from build123d import *

# Parameters (mm, degrees)
SZKIC1_W                    = 80
SZKIC1_H                    = 65
DODANIE_WYCI_GNI_CIE1_DEPTH = 30
SZKIC2_R                    = 27.5
WYTNIJ_WYCI_GNI_CIE1_DEPTH  = 30
SZKIC4_R                    = 3
WYTNIJ_WYCI_GNI_CIE2_DEPTH  = 30
SFAZOWANIE1_SIZE            = 15
SZKIC6_R                    = 3
WYTNIJ_WYCI_GNI_CIE3_DEPTH  = 25
SZKIC8_R                    = 5
WYTNIJ_WYCI_GNI_CIE5_DEPTH  = 6


with BuildPart() as part:
    # Szkic1 → Dodanie-wyciągnięcie1 (new body)
    with BuildSketch(Plane.XY):
        Rectangle(SZKIC1_W, SZKIC1_H)
    extrude(amount=DODANIE_WYCI_GNI_CIE1_DEPTH)

    # Szkic2 → Wytnij-wyciągnięcie1 (cut)
    with BuildSketch(Plane.XY.offset(30)):
        Circle(SZKIC2_R)
    extrude(amount=-WYTNIJ_WYCI_GNI_CIE1_DEPTH, mode=Mode.SUBTRACT)

    # Szkic4 → Wytnij-wyciągnięcie2 (cut)
    with BuildSketch(Plane.XY.offset(30)):
        with Locations((-24, 24)):
            Circle(SZKIC4_R)
        with Locations((24, 24)):
            Circle(SZKIC4_R)
        with Locations((-24, -24)):
            Circle(SZKIC4_R)
        with Locations((24, -24)):
            Circle(SZKIC4_R)
    extrude(amount=-WYTNIJ_WYCI_GNI_CIE2_DEPTH, mode=Mode.SUBTRACT)

    # Sfazowanie1
    sfazowanie1_edges = [part.edges().sort_by_distance(p)[0] for p in [
        (-40, 32.5, 15),
        (40, 32.5, 15),
    ]]
    chamfer(sfazowanie1_edges, length=SFAZOWANIE1_SIZE)

    # Szkic6 → Wytnij-wyciągnięcie3 (cut)
    with BuildSketch(Plane.XZ.offset(32.5)):
        with Locations((-33, 23)):
            Circle(SZKIC6_R)
        with Locations((33, 23)):
            Circle(SZKIC6_R)
        with Locations((33, 7)):
            Circle(SZKIC6_R)
        with Locations((-33, 7)):
            Circle(SZKIC6_R)
    extrude(amount=-WYTNIJ_WYCI_GNI_CIE3_DEPTH, mode=Mode.SUBTRACT)

    # Szkic8 → Wytnij-wyciągnięcie5 (cut)
    with BuildSketch(Plane(origin=(0, 0, 0), x_dir=(-1, 0, 0), z_dir=(0, 0, -1))):
        with Locations((24, -24)):
            Circle(SZKIC8_R)
        with Locations((-24, -24)):
            Circle(SZKIC8_R)
        with Locations((-24, 24)):
            Circle(SZKIC8_R)
        with Locations((24, 24)):
            Circle(SZKIC8_R)
    extrude(amount=-WYTNIJ_WYCI_GNI_CIE5_DEPTH, mode=Mode.SUBTRACT)


solid = part.part
Could you check a few things on this model? Use its own coordinates, in mm. A direction names the side the tool comes from. Round coordinates to 2 decimals unless told otherwise and drop trailing zeros. Loops run counter-clockwise (first coordinate to the right, second up) from the corner with the lowest first, then second, coordinate; pieces in that order, holes last. Notation, with made-up numbers: (-24, -21) -> (17, -21) arc R16 ccw to (17, -11) -> close; hole circle Ø11 at (-23, 50). An arc over 180 degrees is marked (long way). Use CSV: the item, a comma, the result in double quotes.
(1) Suppose I cut it at B-B on y = -24. Write out the boundary of the cut face in (x, z), plus the area to 3 significant figures.
Return value:
outline,"(-40, 0) -> (-29, 0) -> (-29, 6) -> (-27, 6) -> (-27, 30) -> (-40, 30) -> close; (-21, 6) -> (-19, 6) -> (-19, 0) -> (-13.43, 0) -> (-13.43, 30) -> (-21, 30) -> close; (13.43, 0) -> (19, 0) -> (19, 6) -> (21, 6) -> (21, 30) -> (13.43, 30) -> close; (27, 6) -> (29, 6) -> (29, 0) -> (40, 0) -> (40, 30) -> (27, 30) -> close; hole circle Ø6 at (-33, 7); hole circle Ø6 at (-33, 23); hole circle Ø6 at (33, 7); hole circle Ø6 at (33, 23)"
area,"1,070 mm²"
(2) Suppose I cut it at D-D on y = -6. Write out the boundary of the cut face in (x, z).
Return value:
outline,"(-40, 0) -> (-26.84, 0) -> (-26.84, 30) -> (-40, 30) -> close; (26.84, 0) -> (40, 0) -> (40, 30) -> (26.84, 30) -> close"
(3) For faces 4 (the cylindrical face through (30, -20, 7)), 5 (the flat face through (0, 32.5, 15)), 6 (the cylindrical face through (-22.92, 19.12, 2.96)), which set-ups out of +Z, -Z, +X, -X, +Y, -Y let a thin tool reach every point of the face, with its end or its side?
Return value:
face 4,"-Y"
face 5,"+Z, -Z, +X, -X, +Y"
face 6,"-Z"
(4) Will this pin go through, and if not, where does the flat tip stop? pin 1 Ø3.5 at (x, z) = (33, 7) entering from -Y.
Return value:
pin 1,"stops at y = -7.5"
(5) If we mould it in two halves opening along Y, with no side actions, what happens to faces 1 (the cylindrical face through (-20, -27, 3)), 2 (the flat face through (40, -8, 15)), 3 (the flat face through (-1, -32.5, 15))? For each: +Y half, -Y half, draft (parallel to the pull), parting line (faces both ways), or undercut.
Return value:
face 1,"undercut"
face 2,"draft"
face 3,"-Y half"
(6) Suppose I cut it at C-C on x = 18. Write out the boundary of the cut face in (y, z), plus the area to 3 significant figures.
Return value:
outline,"(-32.5, 0) -> (-20.79, 0) -> (-20.79, 30) -> (-32.5, 30) -> close; (20.79, 0) -> (32.5, 0) -> (32.5, 30) -> (20.79, 30) -> close"
area,"703 mm²"
(7) Suppose I cut it at A-A on z = 23. Write out the boundary of the cut face in (x, y).
Return value:
outline,"(-40, -32.5) -> (-36, -32.5) -> (-36, -7.5) -> (-30, -7.5) -> (-30, -32.5) -> (30, -32.5) -> (30, -7.5) -> (36, -7.5) -> (36, -32.5) -> (40, -32.5) -> (40, 17.5) -> (25, 32.5) -> (-25, 32.5) -> (-40, 17.5) -> close; hole circle Ø55 at (0, 0); hole circle Ø6 at (-24, -24); hole circle Ø6 at (-24, 24); hole circle Ø6 at (24, -24); hole circle Ø6 at (24, 24)"
(8) If I drill on probe 1 along Y at (x, z) = (22, 25.75); probe 2 along X at (y, z) = (-20.5, 9.25); probe 3 along Y at (x, z) = (1, 21.25), over which ranges is the centre line in solid material (lowest first)? Write a range as [from, to].
Return value:
probe 1,"y = [-32.5, -26.24], [-21.76, -16.5], [16.5, 21.76], [26.24, 32.5]"
probe 2,"x = [-40, -34.98], [-31.02, -18.33], [18.33, 31.02], [34.98, 40]"
probe 3,"y = [-32.5, -27.48], [27.48, 32.5]"
